Verification items for the finished model (mm, model axes). Face numbers are marked on the shaded views. Coordinates: 2 decimals unless noted, no trailing zeros. Order: outer loops, then holes, each group sorted by start corner. A loop starts at its lowest first (then second) coordinate and runs counter-clockwise, first axis right, second up. Notation, with made-up numbers: M 55,5 L 78,5 A18 ccw 78,28 Z; hole C 27,-17.5 d8. An arc over 180 degrees is marked long. Return JSON: item names as keys, results as strings. Group by question number.
1. Material ranges on line 1 along Z through (x, y) = (44.45, -16) (3 decimals); line 2 along Z through (x, y) = (45.5, -6.5); line 3 along X through (y, z) = (-21.5, 29.5), recorded low to high.
2. Section check A-A, the plane y = -9.75. Give the number of separate pieces and of enclosed holes in the cut face, plus the area to 3 significant figures.
3. Gauge pin test, flat ends, axial feed: pin 1 (5 mm diameter, centred on x = -3.17, z = 40.89, fed in from +Y); pin 2 (8 mm diameter, centred on x = 20.5, y = -6.5, fed in from -Z); pin 3 (6 mm diameter, centred on x = 14.5, y = -7, fed in from -Z); pin 4 (8 mm diameter, centred on y = -9.5, z = 8, fed in from +X). Record the tip position at first contact, or that the pin passes through.
4. Mould release check, pull along Z, two halves, no side actions. Record for the marked faces 1, 2 and 3: +Z half, -Z half, draft (parallel to the pull), parting line (faces both ways), or undercut.
5. Section check C-C, the plane x = 36.5. Record the cut outline in (y, z), plus the area to 3 significant figures.
6. Section check B-B, the plane x = 1.5. Record the cut outline in (y, z).
```python
from build123d import *

# Parameters (mm, degrees)
F0_R     = 3.175
F1_DEPTH = 25.4


with BuildPart() as f1:
    # F0 (on Front) → F1 (new body)
    with BuildSketch(Plane.XZ):
        with BuildLine():
            ThreePointArc((-6.507071, 50.8), (0, 44.292929), (6.507071, 50.8))
            ThreePointArc((6.507071, 50.8), (0, 57.307071), (-6.507071, 50.8))
        make_face()
        with Locations((0, 50.8)):
            Circle(F0_R, mode=Mode.SUBTRACT)
        with BuildLine():
            ThreePointArc((9.2075, 0), (0.211295, 9.205075), (-9.197802, 0.422479))
            ThreePointArc((-9.197802, 0.422479), (-6.658379, -6.359563), (0, -9.2075))
            ThreePointArc((0, -9.2075), (6.510686, -6.510686), (9.2075, 0))
        make_face()
        Circle(F0_R, mode=Mode.SUBTRACT)
        with BuildLine():
            ThreePointArc((54.857703, 0), (51.709039, 7.458327), (44.168189, 10.403887))
            ThreePointArc((44.168189, 10.403887), (34.042297, 0), (44.168189, -10.403887))
            ThreePointArc((44.168189, -10.403887), (51.709039, -7.458327), (54.857703, 0))
        make_face()
        with Locations((44.45, 0)):
            Circle(F0_R, mode=Mode.SUBTRACT)
        with BuildLine():
            Line((7.792568, 30.985557), (6.507071, 50.8))
            ThreePointArc((6.507071, 50.8), (0, 44.292929), (-6.507071, 50.8))
            Line((-6.507071, 50.8), (-7.792568, 30.985557))
            ThreePointArc((-7.792568, 30.985557), (-6.321894, 35.064034), (-2.902509, 37.729493))
            ThreePointArc((-2.902509, 37.729493), (-5.514421, 43.039341), (0, 40.892778))
            ThreePointArc((0, 40.892778), (-0.439454, 39.281128), (-1.636167, 38.115618))
            ThreePointArc((-1.636167, 38.115618), (4.71007, 36.708559), (7.792568, 30.985557))
        make_face()
        with BuildLine():
            ThreePointArc((7.800726, 30.838307), (7.796995, 30.911951), (7.792568, 30.985557))
            ThreePointArc((7.792568, 30.985557), (4.71007, 36.708559), (-1.636167, 38.115618))
            ThreePointArc((-1.636167, 38.115618), (-2.248989, 37.855818), (-2.902509, 37.729493))
            ThreePointArc((-2.902509, 37.729493), (-6.321894, 35.064034), (-7.792568, 30.985557))
            ThreePointArc((-7.792568, 30.985557), (-7.796995, 30.911951), (-7.800726, 30.838307))
            ThreePointArc((-7.800726, 30.838307), (-0.179201, 22.673106), (7.80895, 30.48))
            ThreePointArc((7.80895, 30.48), (7.806894, 30.659201), (7.800726, 30.838307))
        make_face()
        with Locations((0, 30.48)):
            Circle(F0_R, mode=Mode.SUBTRACT)
        with BuildLine():
            Line((8.497322, 15.672671), (7.800726, 30.838307))
            ThreePointArc((7.800726, 30.838307), (7.806894, 30.659201), (7.80895, 30.48))
            ThreePointArc((7.80895, 30.48), (-0.179201, 22.673106), (-7.800726, 30.838307))
            Line((-7.800726, 30.838307), (-9.197802, 0.422479))
            ThreePointArc((-9.197802, 0.422479), (0.211295, 9.205075), (9.2075, 0))
            ThreePointArc((9.2075, 0), (6.510686, -6.510686), (0, -9.2075))
            Line((0, -9.2075), (44.168189, -10.403887))
            ThreePointArc((44.168189, -10.403887), (34.042297, 0), (44.168189, 10.403887))
            Line((44.168189, 10.403887), (15.012092, 9.616351))
            ThreePointArc((15.012092, 9.616351), (10.517129, 11.313251), (8.497322, 15.672671))
        make_face()
    extrude(amount=F1_DEPTH)


solid = f1.part
```
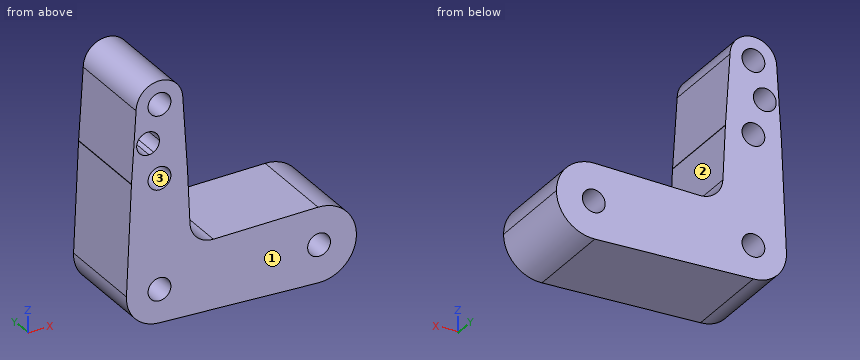
Answers follow:
{
 "1": {"line 1": "-10.408 to -3.175, 3.175 to 10.408", "line 2": "-10.35 to -3, 3 to 10.35", "line 3": "-7.86 to -3.02, 3.02 to 7.86"},
 "2": {"separate pieces": "1", "enclosed holes": "5", "area": "1,750 mm^2"},
 "3": {"pin 1": "through", "pin 2": "z = -9.87", "pin 3": "z = -9.68", "pin 4": "x = 54.06"},
 "4": {"face 1": "draft", "face 2": "+Z half", "face 3": "undercut"},
 "5": {"outline": "M -25.4,-10.2 L 0,-10.2 L 0,10.2 L -25.4,10.2 Z", "area": "518 mm^2"},
 "6": {"outline": "M -25.4,-9.25 L 0,-9.25 L 0,-2.8 L -25.4,-2.8 Z; M -25.4,2.8 L 0,2.8 L 0,27.68 L -25.4,27.68 Z; M -25.4,33.28 L 0,33.28 L 0,48 L -25.4,48 Z; M -25.4,53.6 L 0,53.6 L 0,57.13 L -25.4,57.13 Z"}
}
